Build history of the part. All positions in model axes, mm. Face numbers are marked on the shaded views. A direction names the side the tool comes from. Coordinates: 2 decimals unless noted, no trailing zeros. Order: outer loops, then holes, each group sorted by start corner. A loop starts at its lowest first (then second) coordinate and runs counter-clockwise, first axis right, second up. Notation, with made-up numbers: (-23.75, -31.5) -> (21.25, -31.5) arc R12 ccw to (21.25, -14.5) -> close; hole circle Ø3 at (41.25, 27). An arc over 180 degrees is marked (long way). Write each question's results on one line, items separated by ' | '.
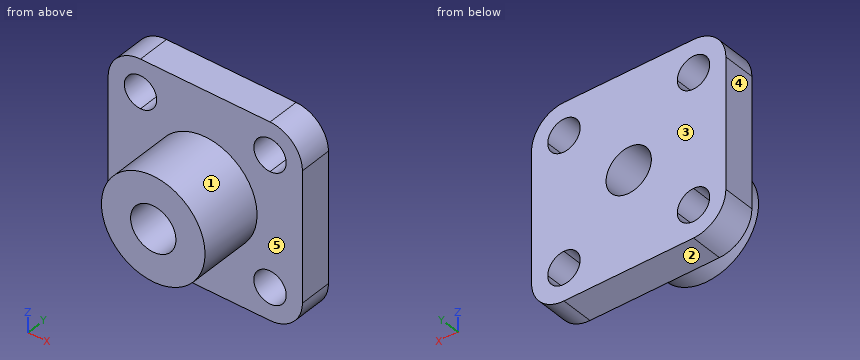
from build123d import *

# Parameters (mm, degrees)
F1_DEPTH = 10
F2_R     = 16
F3_DEPTH = 20
F5_D     = 14


with BuildPart() as f1:
    # F0 (on Front) → F1 (new body)
    with BuildSketch(Plane.XZ):
        with BuildLine():
            ThreePointArc((-16, 0), (0, 16), (16, 0))
            Line((16, 0), (20, 0))
            Line((20, 0), (20, 10))
            ThreePointArc((20, 10), (10, 20), (20, 30))
            Line((20, 30), (-20, 30))
            ThreePointArc((-20, 30), (-12.9289321881, 27.0710678119), (-10, 20))
            ThreePointArc((-10, 20), (-12.9289321881, 12.9289321881), (-20, 10))
            Line((-20, 10), (-20, 0))
            Line((-20, 0), (-16, 0))
        make_face()
        with BuildLine():
            Line((20, 0), (16, 0))
            ThreePointArc((16, 0), (0, -16), (-16, 0))
            Line((-16, 0), (-20, 0))
            Line((-20, 0), (-20, -10))
            ThreePointArc((-20, -10), (-12.9289321881, -12.9289321881), (-10, -20))
            ThreePointArc((-10, -20), (-12.9289321881, -27.0710678119), (-20, -30))
            Line((-20, -30), (20, -30))
            ThreePointArc((20, -30), (10, -20), (20, -10))
            Line((20, -10), (20, 0))
        make_face()
        with BuildLine():
            Line((20, 10), (20, 0))
            Line((20, 0), (20, -10))
            ThreePointArc((20, -10), (27.0710678119, -12.9289321881), (30, -20))
            Line((30, -20), (30, 20))
            ThreePointArc((30, 20), (27.0710678119, 12.9289321881), (20, 10))
        make_face()
        with BuildLine():
            ThreePointArc((20, 30), (10, 20), (20, 10))
            ThreePointArc((20, 10), (27.0710678119, 12.9289321881), (30, 20))
            ThreePointArc((30, 20), (27.0710678119, 27.0710678119), (20, 30))
        make_face()
        with BuildLine():
            ThreePointArc((25, 20), (23.5355339059, 16.4644660941), (20, 15))
            ThreePointArc((20, 15), (16.4644660941, 23.5355339059), (25, 20))
        make_face(mode=Mode.SUBTRACT)
        with BuildLine():
            ThreePointArc((-30, 20), (-27.0710678119, 12.9289321881), (-20, 10))
            ThreePointArc((-20, 10), (-12.9289321881, 12.9289321881), (-10, 20))
            ThreePointArc((-10, 20), (-12.9289321881, 27.0710678119), (-20, 30))
            ThreePointArc((-20, 30), (-27.0710678119, 27.0710678119), (-30, 20))
        make_face()
        with BuildLine():
            ThreePointArc((-15, 20), (-16.4644660941, 16.4644660941), (-20, 15))
            ThreePointArc((-20, 15), (-23.5355339059, 23.5355339059), (-15, 20))
        make_face(mode=Mode.SUBTRACT)
        with BuildLine():
            Line((-20, -10), (-20, 0))
            Line((-20, 0), (-20, 10))
            ThreePointArc((-20, 10), (-27.0710678119, 12.9289321881), (-30, 20))
            Line((-30, 20), (-30, -20))
            ThreePointArc((-30, -20), (-27.0710678119, -12.9289321881), (-20, -10))
        make_face()
        with BuildLine():
            ThreePointArc((-10, -20), (-12.9289321881, -12.9289321881), (-20, -10))
            ThreePointArc((-20, -10), (-27.0710678119, -12.9289321881), (-30, -20))
            ThreePointArc((-30, -20), (-27.0710678119, -27.0710678119), (-20, -30))
            ThreePointArc((-20, -30), (-12.9289321881, -27.0710678119), (-10, -20))
        make_face()
        with BuildLine():
            ThreePointArc((-15, -20), (-23.5355339059, -23.5355339059), (-20, -15))
            ThreePointArc((-20, -15), (-16.4644660941, -16.4644660941), (-15, -20))
        make_face(mode=Mode.SUBTRACT)
        with BuildLine():
            ThreePointArc((30, -20), (27.0710678119, -12.9289321881), (20, -10))
            ThreePointArc((20, -10), (10, -20), (20, -30))
            ThreePointArc((20, -30), (27.0710678119, -27.0710678119), (30, -20))
        make_face()
        with BuildLine():
            ThreePointArc((25, -20), (16.4644660941, -23.5355339059), (20, -15))
            ThreePointArc((20, -15), (23.5355339059, -16.4644660941), (25, -20))
        make_face(mode=Mode.SUBTRACT)
        with BuildLine():
            Line((0, 0), (16, 0))
            ThreePointArc((16, 0), (0, 16), (-16, 0))
            Line((-16, 0), (0, 0))
        make_face()
        with BuildLine():
            ThreePointArc((-16, 0), (0, -16), (16, 0))
            Line((16, 0), (0, 0))
            Line((0, 0), (-16, 0))
        make_face()
    extrude(amount=F1_DEPTH)

    # F2 (on face) → F3 (join)
    with BuildSketch(Plane.XZ.offset(10)):
        Circle(F2_R)
    extrude(amount=F3_DEPTH)

    # F5 (through all)
    with Locations(Plane.XZ.offset(30)):
        with Locations((0, 0)):
            Hole(F5_D / 2)


solid = f1.part
Item 1: Pull direction Y, two halves, no side cores. Call the marked faces 3, 4 and 5: released by +Y, released by -Y, zero draft, split by the parting line, or undercut.
Answer:
face 3: released by +Y | face 4: zero draft | face 5: released by -Y
Item 2: Drill centre lines: line 1 (X direction, y = -5, z = -20); line 2 (Z direction, x = 0, y = -11.25). Where is each one in solid material? Low to high. Write a range as from..to.
Answer:
line 1: x = -30..-25, -15..15, 25..30 | line 2: z = -16..-7, 7..16
Item 3: Slice it at A-A, the plane y = -7. List the corners of the cut face in (x, z), and give its area (3 significant figures).
Answer:
outline: (-30, -20) arc R10 ccw to (-20, -30) -> (20, -30) arc R10 ccw to (30, -20) -> (30, 20) arc R10 ccw to (20, 30) -> (-20, 30) arc R10 ccw to (-30, 20) -> close; hole circle Ø10 at (-20, -20); hole circle Ø10 at (-20, 20); hole circle Ø14 at (0, 0); hole circle Ø10 at (20, -20); hole circle Ø10 at (20, 20) | area: 3,050 mm^2
Item 4: Pin check, flat tips, straight feed: pin 1 (3 mm diameter, centred on x = -10.5, y = -22, fed in from -Z); pin 2 (4 mm diameter, centred on x = 15.5, y = -21, fed in from -Z); pin 3 (6 mm diameter, centred on x = 4, z = 24, fed in from +Y); pin 4 (16 mm diameter, centred on x = 20, z = 20, fed in from -Y). Stop position of each tip, or through.
Answer:
pin 1: stops at z = -13.23 | pin 2: stops at z = -8.59 | pin 3: stops at y = 0 | pin 4: stops at y = -10
Item 5: Slice it at B-B, the plane x = 0. List the corners of the cut face in (y, z).
Answer:
outline: (-30, -16) -> (-10, -16) -> (-10, -30) -> (0, -30) -> (0, -7) -> (-30, -7) -> close; (-30, 7) -> (0, 7) -> (0, 30) -> (-10, 30) -> (-10, 16) -> (-30, 16) -> close
Item 6: Slice it at C-C, the plane x = 21. List the corners of the cut face in (y, z), and give its area (3 significant figures).
Answer:
outline: (-10, -29.95) -> (0, -29.95) -> (0, -24.9) -> (-10, -24.9) -> close; (-10, -15.1) -> (0, -15.1) -> (0, 15.1) -> (-10, 15.1) -> close; (-10, 24.9) -> (0, 24.9) -> (0, 29.95) -> (-10, 29.95) -> close | area: 403 mm^2
Item 7: Tool access for the marked faces 1 and 2: list every direction of +Z, -Z, +X, -X, +Y, -Y with a clear straight run to the whole face (end or side of a thin tool).
Answer:
face 1: -Y | face 2: -Z, +X, -X, +Y, -Y
Item 8: Slice it at D-D, the plane z = 18. List the corners of the cut face in (x, y).
Answer:
outline: (-30, -10) -> (-24.58, -10) -> (-24.58, 0) -> (-30, 0) -> close; (-15.42, -10) -> (15.42, -10) -> (15.42, 0) -> (-15.42, 0) -> close; (24.58, -10) -> (30, -10) -> (30, 0) -> (24.58, 0) -> close
